Job drawing, mm, ordinate dimensions from the low corner. One solid piece. A direction names the side the tool comes from. Give positions to 0.01 mm unless a question says otherwise; leave off trailing zeros. Order: outer loops, then holes, each group sorted by start corner. A loop starts at its lowest first (then second) coordinate and runs counter-clockwise, first axis right, second up. Notation, with made-up numbers: (-28.75, 20) -> (-15.75, 20) arc R37 cw to (-15.75, 57) -> close; hole circle Ø8 at (85, 33.5). An arc over 180 degrees is marked (long way). Use CSV: the item, a comma, the result in double quotes. Start each with the question number.
1. Pull direction Z, two halves, no side cores. Call the marked faces 3 and 4: released by +Z, released by -Z, zero draft, split by the parting line, or undercut.
2. 3-axis set-ups, long thin cutter, end or side, ignore diameter. For the marked faces 1 and 2: which of +Z, -Z, +X, -X, +Y, -Y reach the whole face in a straight line?
3. Drop flat-ended pins along their axis: pin 1 (1 mm diameter, centred on x = 23.47, z = 22.2, fed in from +Y); pin 2 (1 mm diameter, centred on x = 19.5, y = 5.5, fed in from +Z) (1 decimal); pin 3 (2 mm diameter, centred on x = 17, y = 4, fed in from +Z); pin 4 (1.5 mm diameter, centred on x = 18.5, y = 1.5, fed in from +Z). Give the stop position or say it passes through.
4. Cut at D-D on x = 5. List the corners of the cut face in (y, z).
5. Wall check: line 1 (Z direction, x = 7.5, y = 2) (1 decimal); line 2 (X direction, y = 2, z = 3) (1 decimal); line 3 (X direction, y = 1.75, z = 4) (1 decimal). Give the ranges that are in metal, low to high. Write a range as from..to.
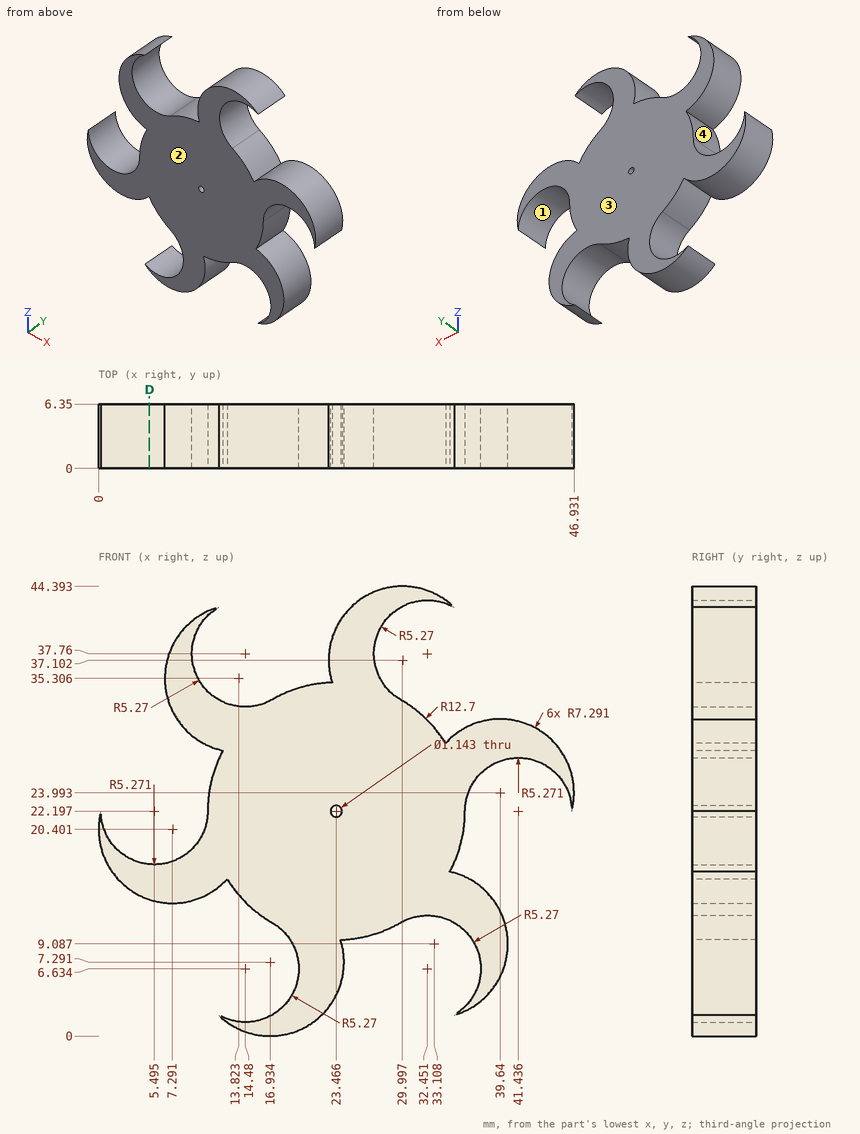
Verdict:
1,face 3,"zero draft"
1,face 4,"undercut"
2,face 1,"+Y, -Y"
2,face 2,"+Z, -Z, +X, -X, -Y"
3,pin 1,"through"
3,pin 2,"z = 34.4"
3,pin 3,"z = 33.66"
3,pin 4,"z = 34.18"
4,outline,"(0, 13.48) -> (6.35, 13.48) -> (6.35, 16.95) -> (0, 16.95) -> close"
5,line 1,"13.1..17.3, 31.7..38.9"
5,line 2,"18.3..22.8, 36.3..37.1"
5,line 3,"19..23.4, 37..38.3"
